The model under review builds one solid part; all positions refer to its coordinate system, in mm. A direction names the side the tool comes from. Give positions to 0.01 mm unless a question says otherwise; leave off trailing zeros. Order: outer loops, then holes, each group sorted by start corner. A loop starts at its lowest first (then second) coordinate and runs counter-clockwise, first axis right, second up.
```python
from build123d import *

# Parameters (mm, degrees)
EXTRUSION1_DEPTH = 5


with BuildPart() as part:
    # Esquisse1 → Révolution1 (revolve)
    with BuildSketch(Plane.XY, mode=Mode.PRIVATE) as r_volution1_sk:
        with BuildLine():
            Line((-12, 5), (-12, 8))
            ThreePointArc((-12, 8), (-8.192021355, 8.387659794), (-5, 10.5))
            Line((-5, 10.5), (-4, 10.5))
            Line((-4, 10.5), (-4, 13.5))
            Line((-4, 13.5), (0, 13.5))
            Line((0, 13.5), (0, 5))
            Line((0, 5), (-12, 5))
        make_face()
    revolve(r_volution1_sk.sketch.rotate(Axis((-16.08577031, 0, 0), (1, 0, 0)), 90), axis=Axis((-16.08577031, 0, 0), (1, 0, 0)))  # turned: the seam where the file's is

    # Esquisse2 → Extrusion1 (add)
    with BuildSketch(Plane(origin=(0, 0, 0), x_dir=(0, 0, -1), z_dir=(1, 0, 0))):
        with BuildLine():
            Line((-5, 12.539936204), (-5, 3.31662479))
            ThreePointArc((-5, 3.31662479), (0, 6), (5, 3.31662479))
            Line((5, 3.31662479), (5, 12.539936204))
            ThreePointArc((5, 12.539936204), (0, 13.5), (-5, 12.539936204))
        make_face()
    extrude(amount=EXTRUSION1_DEPTH)


solid = part.part
```
Item 1: Take a section at A-A (z = 0). Give the boundary of the cut face in (x, y).
Values found:
outline: (-12, -8) arc R8 cw to (-5, -10.5) - (-4, -10.5) - (-4, -13.5) - (0, -13.5) - (0, -5) - (-12, -5) - close; (-12, 5) - (0, 5) - (0, 6) - (5, 6) - (5, 13.5) - (-4, 13.5) - (-4, 10.5) - (-5, 10.5) arc R8 cw to (-12, 8) - close
Item 2: For line 1 (Y direction, x = -0.5, z = 0.25); line 2 (X direction, y = 8.75, z = 7.5); line 3 (Y direction, x = -5.5, z = -4.5), list the stretches that pass through material, from the lowest coordinate up.
Values found:
line 1: y = -13.5 to -4.99, 4.99 to 13.5
line 2: x = -4 to 0
line 3: y = -8.93 to -2.18, 2.18 to 8.93
Item 3: Take a section at D-D (x = 3.75). Give the boundary of the cut face in (y, z).
Values found:
outline: (3.32, -5) - (12.54, -5) arc R13.5 ccw to (12.54, 5) - (3.32, 5) arc R6 cw to start
Item 4: Take a section at C-C (x = -3.5). Give the boundary of the cut face in (y, z), and give its area (3 significant figures).
Values found:
outline: circle Ø27 at (0, 0); hole circle Ø10 at (0, 0)
area: 494 mm2
Item 5: Clearance check with flat-ended pins moving along their axes: pin 1 Ø10 at (x, y) = (1.5, 5.5) entering from +Z; pin 2 Ø1.5 at (x, z) = (-4, -5.5) entering from +Y; pin 3 Ø2 at (x, z) = (-4.5, 0) entering from +Y; pin 4 Ø2.5 at (x, y) = (3.5, 9.5) entering from +Z. State where each tip first meets the part, or that it passes through.
Values found:
pin 1: stops at z = 13.48
pin 2: stops at y = 12.64
pin 3: stops at y = 13.5
pin 4: stops at z = 5
Item 6: Take a section at B-B (y = 0). Give the boundary of the cut face in (x, z).
Values found:
outline: (-12, -8) arc R8 cw to (-5, -10.5) - (-4, -10.5) - (-4, -13.5) - (0, -13.5) - (0, -5) - (-12, -5) - close; (-12, 5) - (0, 5) - (0, 13.5) - (-4, 13.5) - (-4, 10.5) - (-5, 10.5) arc R8 cw to (-12, 8) - close
Item 7: Draft analysis for pull direction Z (two halves, no side actions). For faces 5 (the cylindrical face through (2, 6, 0)), 6 (the flat face through (-12, -0.1, -5.2)), 7 (the cylindrical face through (-6, 0, -5)), 8 (the cylindrical face through (-4.5, -3.2, 10)), state which applies: released by +Z, released by -Z, zero draft, split by the parting line, or undercut.
Values found:
face 5: undercut
face 6: zero draft
face 7: undercut
face 8: split by the parting line
Item 8: For faces 1 (the flat face through (2, 8, -5)), 2 (the flat face through (-4, 11, 0)), 3 (the flat face through (5, 10, 0)), 4 (the flat face through (2, 8, 5)), list the 3-axis set-ups (+Z, -Z, +X, -X, +Y, -Y) from which the entire face can be reached by the end or side of a thin tool; tool diameter is ignored.
Values found:
face 1: -Z, +X, +Y, -Y
face 2: -X
face 3: +Z, -Z, +X, +Y, -Y
face 4: +Z, +X, +Y, -Y
